Could you check a few things on this model? Use its own coordinates, in mm. A direction names the side the tool comes from. Coordinates: 2 decimals unless noted, no trailing zeros. Loops run counter-clockwise (first coordinate to the right, second up) from the corner with the lowest first, then second, coordinate; pieces in that order, holes last. Notation, with made-up numbers: (-11, 50.5) - (6, 50.5) arc R11 cw to (6, 57.5) - close; hole circle Ø5 at (25, 3.5). An arc over 180 degrees is marked (long way). One line per question, with ' | ' between items. Start each with the question number.
1. I want a section at D-D, the plane z = -8.5. Write out the boundary of the cut face in (x, y).
2. I'm going to push flat-ended pins straight in: P1, Ø13, axis at x = 0, z = 0, coming from the +Y side; P2, Ø10, axis at x = -21.5, z = 1, coming from the +Y side; P3, Ø1.8, axis at x = -18, y = 6, coming from the +Z side. Where does each tip first touch, or does it pass through?
3. I want a section at B-B, the plane x = -8. Write out the boundary of the cut face in (y, z).
4. Please list where these lines run through material, in increasing order: L1, parallel to X at y = 1.2, z = 0; L2, parallel to Y at x = 22.5, z = 0; L3, parallel to Z at x = 3, y = 2.25. Write a range as [from, to].
5. I want a section at C-C, the plane y = 8.25. Write out the boundary of the cut face in (x, z), then the cut area to 3 significant figures.
6. Which directions (+Z, -Z, +X, -X, +Y, -Y) give clear straight access to the entire face, cutting with the end or side of a thin tool? Please do faces 1 (the cylindrical face through (-10.74, 7.45, -2.38)), 2 (the flat face through (-18, 6, 4.5)), 3 (the flat face through (18, 6, 4.5)), 4 (the cylindrical face through (-7.576, 1.972, -9.88)).
7. I want a section at A-A, the plane z = 0. Write out the boundary of the cut face in (x, y).
from build123d import *

# Parameters (mm, degrees)
SKETCH1_R           = 12.45
SKETCH1_R_2         = 6
BOSS_EXTRUDE1_DEPTH = 4
SKETCH2_R           = 16
SKETCH2_R_2         = 11
BOSS_EXTRUDE2_DEPTH = 7
BOSS_EXTRUDE3_START = -7
SKETCH3_R           = 1.55
BOSS_EXTRUDE3_DEPTH = 3.5
CIRPATTERN1_COUNT   = 4


with BuildPart() as part:
    # Sketch1 → Boss-Extrude1 (new body)
    with BuildSketch(Plane(origin=(0, 0, 0), x_dir=(1, 0, 0), z_dir=(0, 1, 0))):
        with Locations(Location((0, 0, 0), (0, 0, 270))):
            Circle(SKETCH1_R)
        with Locations(Location((0, 0, 0), (0, 0, 270))):
            Circle(SKETCH1_R_2, mode=Mode.SUBTRACT)
    extrude(amount=BOSS_EXTRUDE1_DEPTH)

    # Sketch2 → Boss-Extrude2 (add)
    with BuildSketch(Plane(origin=(0, 4, 0), x_dir=(1, 0, 0), z_dir=(0, 1, 0))):
        with Locations(Location((0, 0, 0), (0, 0, 270))):
            Circle(SKETCH2_R)
        with Locations(Location((0, 0, 0), (0, 0, 270))):
            Circle(SKETCH2_R_2, mode=Mode.SUBTRACT)
    extrude(amount=BOSS_EXTRUDE2_DEPTH)

    # Sketch3 → Boss-Extrude3 (add)
    with BuildSketch(Plane(origin=(0, 11, 0), x_dir=(1, 0, 0), z_dir=(0, 1, 0)).offset(BOSS_EXTRUDE3_START)):
        with BuildLine():
            Line((-4.5, 20), (-4.5, 15.354152533))
            ThreePointArc((-4.5, 15.354152533), (0, 16), (4.5, 15.354152533))
            Line((4.5, 15.354152533), (4.5, 20))
            ThreePointArc((4.5, 20), (0, 24.5), (-4.5, 20))
        make_face()
        with Locations(Location((0, 20, 0), (0, 0, 270))):
            Circle(SKETCH3_R, mode=Mode.SUBTRACT)
    boss_extrude3 = extrude(amount=BOSS_EXTRUDE3_DEPTH)

    # CirPattern1: Boss-Extrude3 ×4 about axis
    cirpattern1_axis = Axis((0, 0, 0), (0, 1, 0))
    for i in range(1, CIRPATTERN1_COUNT):
        add(boss_extrude3.rotate(cirpattern1_axis, i * 360 / CIRPATTERN1_COUNT))


solid = part.part
Results are:
1) outline: (-13.56, 4) - (-9.1, 4) - (-9.1, 0) - (9.1, 0) - (9.1, 4) - (13.56, 4) - (13.56, 11) - (6.98, 11) - (6.98, 4) - (-6.98, 4) - (-6.98, 11) - (-13.56, 11) - close
2) P1: stops at y = 4 | P2: stops at y = 7.5 | P3: stops at z = 4.5
3) outline: (0, -9.54) - (4, -9.54) - (4, -13.86) - (11, -13.86) - (11, -7.55) - (4, -7.55) - (4, 7.55) - (11, 7.55) - (11, 13.86) - (4, 13.86) - (4, 9.54) - (0, 9.54) - close
4) L1: x = [-12.45, -6], [6, 12.45] | L2: y = [4, 7.5] | L3: z = [-12.08, -5.2], [5.2, 12.08]
5) outline: circle Ø32 at (0, 0); hole circle Ø22 at (0, 0) | area: 424 mm2
6) face 1: +Y | face 2: +Z, -X, +Y, -Y | face 3: +Z, +X, +Y, -Y | face 4: -Y
7) outline: (-24.5, 4) - (-21.55, 4) - (-21.55, 7.5) - (-24.5, 7.5) - close; (-18.45, 4) - (-12.45, 4) - (-12.45, 0) - (-6, 0) - (-6, 4) - (-11, 4) - (-11, 11) - (-16, 11) - (-16, 7.5) - (-18.45, 7.5) - close; (6, 0) - (12.45, 0) - (12.45, 4) - (18.45, 4) - (18.45, 7.5) - (16, 7.5) - (16, 11) - (11, 11) - (11, 4) - (6, 4) - close; (21.55, 4) - (24.5, 4) - (24.5, 7.5) - (21.55, 7.5) - close
